Could you check a few things on this drawing? It's one solid part, dimensions in mm from its lowest x, y, z. A direction names the side the tool comes from. Give positions to 0.01 mm unless a question says otherwise; leave off trailing zeros. Order: outer loops, then holes, each group sorted by start corner. A loop starts at its lowest first (then second) coordinate and runs counter-clockwise, first axis right, second up.
Item 1: I want a section at A-A, the plane y = 30. Count the separate pieces of the cut face and the enclosed holes in it, then the cut area to 3 significant figures.
Item 2: If I drill on line 1 along Z through (x, y) = (511.5, 28); line 2 along Y through (x, z) = (21, 112); line 3 along X through (y, z) = (40, 346.5), over which ranges is the centre line in solid material (lowest first)?
Item 3: I want a section at D-D, the plane x = 21.15. Write out the boundary of the cut face in (y, z), then the cut area to 3 significant figures.
Item 4: Which directions (+Z, -Z, +X, -X, +Y, -Y) give clear straight access to the entire face, cutting with the end or side of a thin tool? Please do the marked faces 1, 2 and 3.
Item 5: I want a section at C-C, the plane x = 555. Write out the boundary of the cut face in (y, z), then the cut area to 3 significant figures.
Item 6: I want a section at B-B, the plane z = 313.5. Write out the boundary of the cut face in (x, y), then the cut area to 3 significant figures.
Item 7: If we mould it in two halves opening along Z, with no side actions, what happens to the marked faces 4, 5 and 6? For each: +Z half, -Z half, draft (parallel to the pull), parting line (faces both ways), or undercut.
Item 8: I'm going to push flat-ended pins straight in: pin 1 Ø18 at (x, y) = (555.5, 16.5) entering from -Z; pin 2 Ø8 at (y, z) = (15, 188) entering from +X. Where does each tip first touch, or does it pass through?
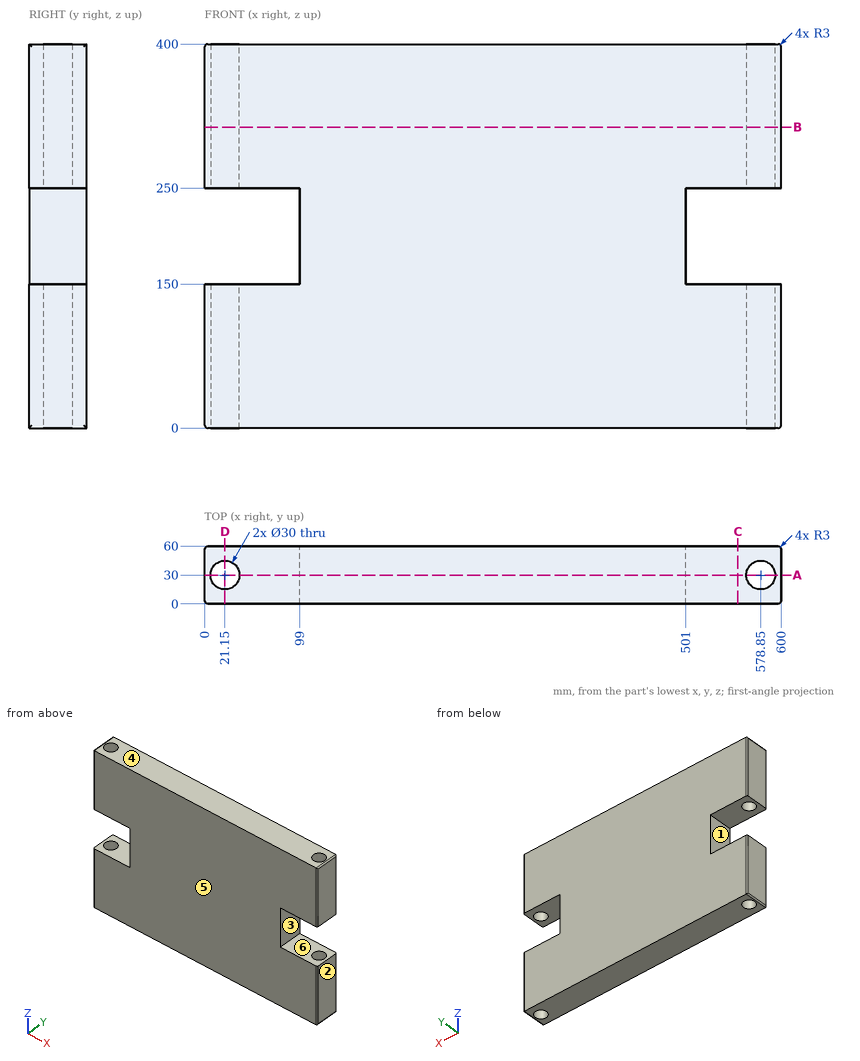
Results list:
1. separate pieces: 5
1. enclosed holes: 0
1. area: 202,000 mm2
2. line 1: z = 0 to 150, 250 to 400
2. line 2: y = 0 to 15, 45 to 60
2. line 3: x = 0 to 9.97, 32.33 to 567.67, 590.03 to 600
3. outline: (0, 0) - (15, 0) - (15, 150) - (0, 150) - close; (0, 250) - (15, 250) - (15, 400) - (0, 400) - close; (45, 0) - (60, 0) - (60, 150) - (45, 150) - close; (45, 250) - (60, 250) - (60, 400) - (45, 400) - close
3. area: 9,000 mm2
4. face 1: -X, +Y, -Y
4. face 2: +Z, -Z, +X, +Y, -Y
4. face 3: +X, +Y, -Y
5. outline: (0, 0) - (60, 0) - (60, 150) - (0, 150) - close; (0, 250) - (60, 250) - (60, 400) - (0, 400) - close
5. area: 18,000 mm2
6. outline: (0, 3) arc R3 ccw to (3, 0) - (597, 0) arc R3 ccw to (600, 3) - (600, 57) arc R3 ccw to (597, 60) - (3, 60) arc R3 ccw to (0, 57) - close; hole circle Ø30 at (21.15, 30); hole circle Ø30 at (578.85, 30)
6. area: 34,600 mm2
7. face 4: +Z half
7. face 5: draft
7. face 6: undercut
8. pin 1: stops at z = 0
8. pin 2: stops at x = 501
